The listing builds one solid part. Answer for the finished solid, in the listing's coordinates (mm). A direction names the side the tool comes from. Round coordinates to 2 decimals unless told otherwise and drop trailing zeros. Loops run counter-clockwise (first coordinate to the right, second up) from the corner with the lowest first, then second, coordinate; pieces in that order, holes last. Notation, with made-up numbers: (83, 49.5) -> (134, 49.5) arc R20 ccw to (134, 74.5) -> close; hole circle Ø8 at (-30, 44.5). An arc over 180 degrees is marked (long way). One line per question, with ' | ' between items.
from build123d import *

# Parameters (mm, degrees)
SKETCH_W              = 115
SKETCH_H              = 25
PAD_DEPTH             = 3
PAD001_DEPTH          = 3
SKETCH002_W           = 115
SKETCH002_H           = 25
SKETCH002_W_2         = 96.5
SKETCH002_H_2         = 3
PAD002_DEPTH          = 3
SKETCH003_R           = 1.55
POCKET_DEPTH          = 245.060315
POLARPATTERN_COUNT    = 2
POLARPATTERN001_COUNT = 2
POLARPATTERN002_COUNT = 2
FILLET_R              = 2


with BuildPart() as part:
    # Sketch → Pad (new body)
    with BuildSketch(Plane.XY):
        Rectangle(SKETCH_W, SKETCH_H)
    extrude(amount=PAD_DEPTH)

    # Sketch001 (on Face6 of Pad) → Pad001 (join)
    with BuildSketch(Plane.XY.offset(3)):
        Polygon((-57.5, 12.5), (57.5, 12.5), (57.5, 4), (50, 4), (50, 5), (-50, 5), (-50, 4), (-57.5, 4), align=None)
        Polygon((-57.5, -12.5), (57.5, -12.5), (57.5, -4), (50, -4), (50, -5), (-50, -5), (-50, -4), (-57.5, -4), align=None)
    extrude(amount=PAD001_DEPTH)

    # Sketch002 (on Face12 of Pad001) → Pad002 (join)
    with BuildSketch(Plane.XY.offset(6)):
        Rectangle(SKETCH002_W, SKETCH002_H)
        Rectangle(SKETCH002_W_2, SKETCH002_H_2, mode=Mode.SUBTRACT)
    extrude(amount=PAD002_DEPTH)

    # Sketch003 (on Face26 of Pad002) → Pocket (cut, through all)
    with BuildSketch(Plane.XY.offset(9)):
        with Locations((-52.5, 7.5)):
            Circle(SKETCH003_R)
    pocket = extrude(amount=-POCKET_DEPTH, mode=Mode.SUBTRACT)

    # PolarPattern: Pocket ×2 about axis
    polarpattern_axis = Axis((0, 0, 0), (0, 1, 0))
    for i in range(1, POLARPATTERN_COUNT):
        add(pocket.rotate(polarpattern_axis, i * 360 / POLARPATTERN_COUNT), mode=Mode.SUBTRACT)

    # PolarPattern001: Pocket ×2 about axis
    polarpattern001_axis = Axis((0, 0, 0), (1, 0, 0))
    for i in range(1, POLARPATTERN001_COUNT):
        add(pocket.rotate(polarpattern001_axis, i * 360 / POLARPATTERN001_COUNT), mode=Mode.SUBTRACT)

    # PolarPattern002: Pocket ×2 about axis
    polarpattern002_axis = Axis((0, 0, 9), (0, 0, 1))
    for i in range(1, POLARPATTERN002_COUNT):
        add(pocket.rotate(polarpattern002_axis, i * 360 / POLARPATTERN002_COUNT), mode=Mode.SUBTRACT)

    # Fillet
    fillet_edges = [part.edges().sort_by_distance(p)[0] for p in [
        (57.5, 12.5, 7.5),
        (57.5, 12.5, 4.5),
        (57.5, 12.5, 1.5),
        (57.5, -12.5, 7.5),
        (-57.5, 12.5, 7.5),
        (-57.5, -12.5, 7.5),
    ]]
    fillet(fillet_edges, radius=FILLET_R)


solid = part.part
Q1. A cutting plane is placed at B-B on y = 2.5. Give the vertices of the cut face in (x, z), plus the area to 3 significant figures.
Numbers:
outline: (-57.5, 0) -> (57.5, 0) -> (57.5, 3) -> (-57.5, 3) -> close; (-57.5, 6) -> (57.5, 6) -> (57.5, 9) -> (-57.5, 9) -> close | area: 690 mm^2
Q2. Find the intervals of material crossed by line 1 (X direction, y = -7.5, z = 5.25); line 2 (Y direction, x = 52.5, z = 5.5); line 3 (Y direction, x = 52.5, z = 2), in increasing order. Write a range as from..to.
Numbers:
line 1: -57.5..-54.05, -50.95..50.95, 54.05..57.5 | line 2: -12.5..-9.05, -5.95..-4, 4..5.95, 9.05..12.5 | line 3: -12.5..-9.05, -5.95..5.95, 9.05..12.5
Q3. For a pull along X with two mould halves and no side action, classify faces 5 (the face through (-1, 3, 9)), 6 (the face through (-1, -1.5, 7)), 7 (the face through (-57.5, -0.1, 6.4)), 8 (the face through (56.9, 11.93, 4.44)) as pulls with the +X half, pulls with the -X half, needs draft (parallel to the pull), parting line crosses it, or undercut.
Numbers:
face 5: needs draft | face 6: undercut | face 7: pulls with the -X half | face 8: pulls with the +X half
Q4. A cutting plane is placed at C-C on y = -7.5. Give the vertices of the cut face in (x, z).
Numbers:
outline: (-57.5, 0) -> (-54.05, 0) -> (-54.05, 9) -> (-57.5, 9) -> close; (-50.95, 0) -> (50.95, 0) -> (50.95, 9) -> (-50.95, 9) -> close; (54.05, 0) -> (57.5, 0) -> (57.5, 9) -> (54.05, 9) -> close
Q5. A cutting plane is placed at A-A on x = 52.5. Give the vertices of the cut face in (y, z), plus the area to 3 significant figures.
Numbers:
outline: (-12.5, 0) -> (-9.05, 0) -> (-9.05, 9) -> (-12.5, 9) -> close; (-5.95, 0) -> (5.95, 0) -> (5.95, 9) -> (-5.95, 9) -> close; (9.05, 0) -> (12.5, 0) -> (12.5, 9) -> (9.05, 9) -> close; hole (-4, 3) -> (4, 3) -> (4, 6) -> (-4, 6) -> close | area: 145 mm^2
Q6. For faces 1 (the face through (57.5, -0.1, 6.4)), 2 (the face through (54, -4, 4)), 3 (the face through (-48.25, 0, 7)), 4 (the face through (-1, 0, 3)), determine the directions among +Z, -Z, +X, -X, +Y, -Y from which every point of the face is accessible in a straight line to the end or side of a thin tool.
Numbers:
face 1: +Z, -Z, +X, +Y, -Y | face 2: +X, -X | face 3: +Z | face 4: none
Q7. A cutting plane is placed at D-D on z = 7.25. Give the vertices of the cut face in (x, y), plus the area to 3 significant figures.
Numbers:
outline: (-57.5, -10.5) arc R2 ccw to (-55.5, -12.5) -> (55.5, -12.5) arc R2 ccw to (57.5, -10.5) -> (57.5, 10.5) arc R2 ccw to (55.5, 12.5) -> (-55.5, 12.5) arc R2 ccw to (-57.5, 10.5) -> close; hole circle Ø3.1 at (-52.5, -7.5); hole circle Ø3.1 at (-52.5, 7.5); hole (-48.25, -1.5) -> (48.25, -1.5) -> (48.25, 1.5) -> (-48.25, 1.5) -> close; hole circle Ø3.1 at (52.5, -7.5); hole circle Ø3.1 at (52.5, 7.5) | area: 2,550 mm^2
